Can you work these out from the drawing? Everything is in mm from the part's minimum corner. Coordinates: 2 decimals unless noted, no trailing zeros. Order: outer loops, then holes, each group sorted by start corner. A loop starts at its lowest first (then second) coordinate and runs counter-clockwise, first axis right, second up. Notation, with made-up numbers: (83, 13) - (138, 13) arc R25 cw to (138, 51) - close; hole circle Ø6 at (-31, 84). An arc over 180 degrees is marked (long way). Use one line per item in the form item = value. Start each with the question number.
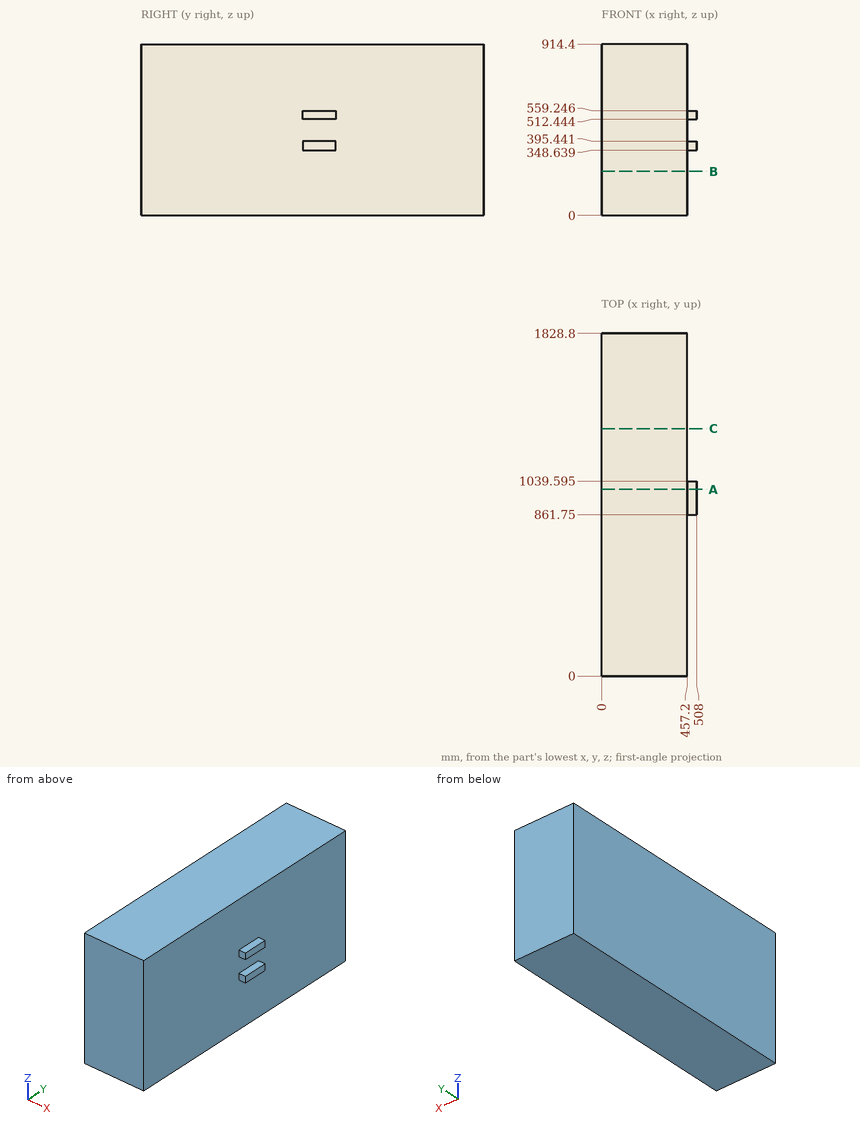
1) Suppose I cut it at C-C, the plane y = 1320. List the corners of the cut face in (x, z) for me, then the cut area to 3 significant figures.
2) For pin 1 (23.5 mm diameter, centred on x = 493, z = 370, fed in from -Y), with a flat end and sliding along its axis, tell me the tip position at first contact or that it passes through.
3) Suppose I cut it at A-A, the plane y = 996. List the corners of the cut face in (x, z) for me (1 decimal).
4) I need wall thicknesses on probe 1 along X at (y, z) = (749.5, 140). Which ranges of the line are inside material? Lowest first, please. Write a range as [from, to].
5) Suppose I cut it at B-B, the plane z = 235. List the corners of the cut face in (x, y) for me, then the cut area to 3 significant figures.
From the geometry:
q1.outline = (0, 0) - (457.2, 0) - (457.2, 914.4) - (0, 914.4) - close
q1.area = 418,000 mm2
q2.pin_1 = 861.75
q3.outline = (0, 0) - (457.2, 0) - (457.2, 348.6) - (508, 348.6) - (508, 395.4) - (457.2, 395.4) - (457.2, 512.4) - (508, 512.4) - (508, 559.2) - (457.2, 559.2) - (457.2, 914.4) - (0, 914.4) - close
q4.probe_1 = [0, 457.2]
q5.outline = (0, 0) - (457.2, 0) - (457.2, 1828.8) - (0, 1828.8) - close
q5.area = 836,000 mm2
